```python
from build123d import *


with BuildPart() as part:
    # 草图1 → 旋转1 (revolve)
    with BuildSketch(Plane(origin=(0, 0, 0), x_dir=(0, 0, -1), z_dir=(1, 0, 0)), mode=Mode.PRIVATE) as revolve_1_sk:
        with BuildLine():
            Line((33, 0), (33, -5))
            Line((33, -5), (35.5, -5))
            Line((35.5, -5), (35.5, -36))
            ThreePointArc((35.5, -36), (34.914213562, -37.414213562), (33.5, -38))
            Line((33.5, -38), (0, -38))
            Line((0, -38), (0, -37))
            Line((0, -37), (33.5, -37))
            ThreePointArc((33.5, -37), (34.207106781, -36.707106781), (34.5, -36))
            Line((34.5, -36), (34.5, -6))
            Line((34.5, -6), (32, -6))
            Line((32, -6), (32, 0))
            Line((32, 0), (33, 0))
        make_face()
    revolve(revolve_1_sk.sketch.rotate(Axis((0, 1.9, 0), (0, -1, 0)), 180), axis=Axis((0, 1.9, 0), (0, -1, 0)))


solid = part.part
```
CAD build for the part. Positions are in the model's coordinates, mm. A direction names the side the tool comes from. Coordinates: 2 decimals unless noted, no trailing zeros. Order: outer loops, then holes, each group sorted by start corner. A loop starts at its lowest first (then second) coordinate and runs counter-clockwise, first axis right, second up. Notation, with made-up numbers: (-36.5, -32) - (-5.5, -32) arc R21 ccw to (-5.5, -25) - close; hole circle Ø6 at (-3.75, 17). An arc over 180 degrees is marked (long way). Answer in a Markdown table with one row per item.
1. Slice it at C-C, the plane y = -3. List the corners of the cut face in (x, z).
Answer:
| item | result |
|---|---|
| outline | circle Ø66 at (0, 0); hole circle Ø64 at (0, 0) |
2. Slice it at A-A, the plane x = 0. List the corners of the cut face in (y, z), then the cut area to 3 significant figures.
Answer:
| item | result |
|---|---|
| outline | (-38, -33.5) arc R2 ccw to (-36, -35.5) - (-5, -35.5) - (-5, -33) - (0, -33) - (0, -32) - (-6, -32) - (-6, -34.5) - (-36, -34.5) arc R1 cw to (-37, -33.5) - (-37, 33.5) arc R1 cw to (-36, 34.5) - (-6, 34.5) - (-6, 32) - (0, 32) - (0, 33) - (-5, 33) - (-5, 35.5) - (-36, 35.5) arc R2 ccw to (-38, 33.5) - close |
| area | 149 mm² |
3. Drill centre lines: L1, parallel to X at y = -4, z = 0; L2, parallel to X at y = -17.5, z = 0; L3, parallel to Y at x = -9, z = 32. Where is each one in solid material? Low to high. Write a range as from..to.
Answer:
| item | result |
|---|---|
| L1 | -33..-32, 32..33 |
| L2 | -35.5..-34.5, 34.5..35.5 |
| L3 | -38..-37, -6..-5 |
4. Flat gauge pins, fed straight in: P1, Ø4, axis at x = -17.5, y = -21, coming from the -Z side; P2, Ø10, axis at x = 7, y = -26.5, coming from the -Z side; P3, Ø1, axis at x = -25.5, z = 12.5, coming from the +Y side. Where does each tip first touch, or does it go through?
Answer:
| item | result |
|---|---|
| P1 | z = -31.94 |
| P2 | z = -35.44 |
| P3 | y = -37 |
5. Slice it at B-B, the plane z = 0. List the corners of the cut face in (x, y), then the cut area to 3 significant figures.
Answer:
| item | result |
|---|---|
| outline | (-35.5, -36) arc R2 ccw to (-33.5, -38) - (33.5, -38) arc R2 ccw to (35.5, -36) - (35.5, -5) - (33, -5) - (33, 0) - (32, 0) - (32, -6) - (34.5, -6) - (34.5, -36) arc R1 cw to (33.5, -37) - (-33.5, -37) arc R1 cw to (-34.5, -36) - (-34.5, -6) - (-32, -6) - (-32, 0) - (-33, 0) - (-33, -5) - (-35.5, -5) - close |
| area | 149 mm² |
6. Slice it at D-D, the plane y = -17. List the corners of the cut face in (x, z).
Answer:
| item | result |
|---|---|
| outline | circle Ø71 at (0, 0); hole circle Ø69 at (0, 0) |
7. Pull direction Z, two halves, no side cores. Call faces 4 (the face through (34.656, -20.717, -7.696)), 5 (the face through (31, -6, 10)), 6 (the face through (24, -5, -24)): +Z half, -Z half, draft (parallel to the pull), parting line (faces both ways), or undercut.
Answer:
| item | result |
|---|---|
| face 4 | parting line |
| face 5 | undercut |
| face 6 | draft |
8. 3-axis set-ups, long thin cutter, end or side, ignore diameter. For faces 1 (the face through (0, -38, 0)), 2 (the face through (-1.517, -20.79, -34.467)), 3 (the face through (-9.912, -2.535, 31.476)): which of +Z, -Z, +X, -X, +Y, -Y reach the whole face in a straight line?
Answer:
| item | result |
|---|---|
| face 1 | +Z, -Z, +X, -X, -Y |
| face 2 | none |
| face 3 | +Y |
